Geometry check sheet. Reference: drawing and pictorial views, mm from the part's lowest x, y, z. Give positions to 0.01 mm unless a question says otherwise; leave off trailing zeros. Write each loop counter-clockwise with the first axis right and the second up, starting at its lowest first coordinate (ties: lowest second). Pieces come first, ordered by that corner, then holes. Notation, with made-up numbers: (22.25, 3) - (37.25, 3) arc R13 cw to (37.25, 17) - close; hole circle Ø5 at (23, 81.25). An arc over 180 degrees is marked (long way). Put each result on its own line as item: value.
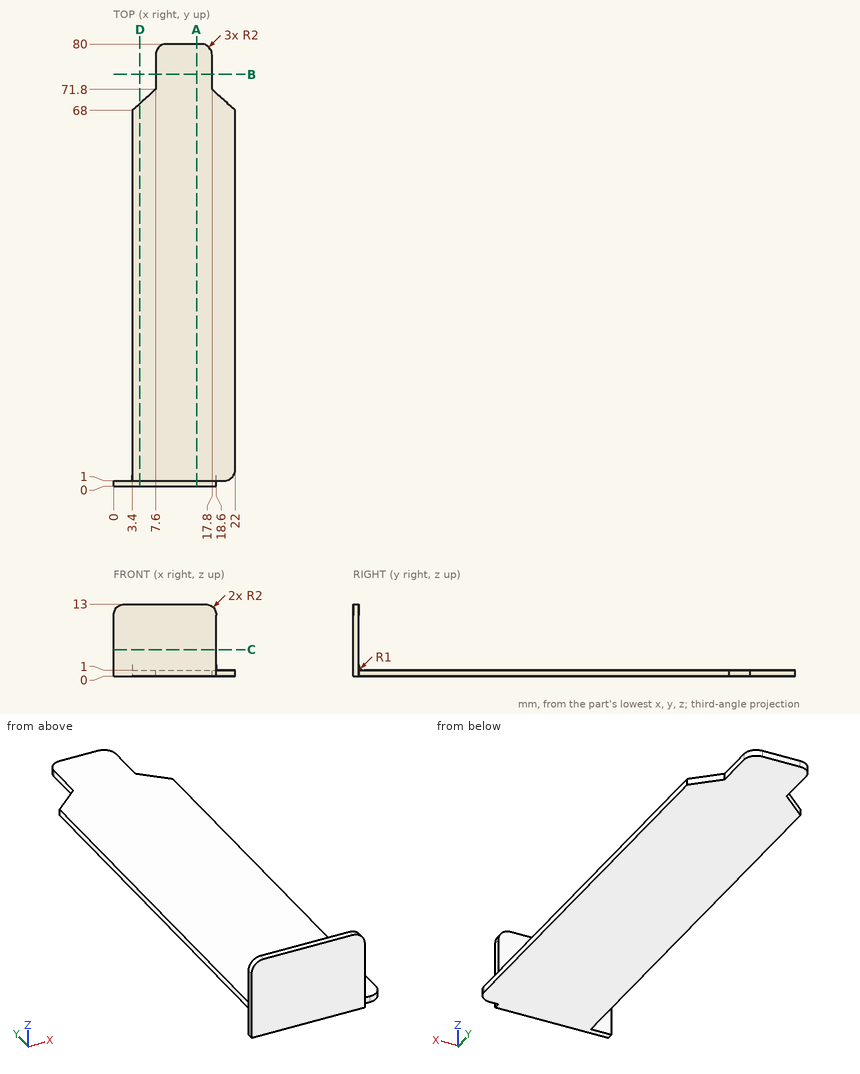
Q1. Section check D-D, the plane x = 4.75. Record the cut outline in (y, z).
Answers follow:
outline: (0, 0) - (69.22, 0) - (69.22, 1) - (2, 1) arc R1 cw to (1, 2) - (1, 13) - (0, 13) - close
Q2. Go/stop test with flat-tipped pins: pin 1 Ø1.1 at (y, z) = (75.5, 0.5) entering from -X; pin 2 Ø2 at (y, z) = (32, 1) entering from -X; pin 3 Ø5.5 at (x, y) = (13.5, 46.5) entering from +Z. Record where each tip stops, or that it passes through.
Answers follow:
pin 1: stops at x = 7.6
pin 2: stops at x = 3.4
pin 3: stops at z = 1
Q3. Section check A-A, the plane x = 15. Record the cut outline in (y, z), plus the area to 3 significant figures.
Answers follow:
outline: (0, 0) - (80, 0) - (80, 1) - (2, 1) arc R1 cw to (1, 2) - (1, 13) - (0, 13) - close
area: 92.2 mm2
Q4. Section check C-C, the plane z = 4.75. Record the cut outline in (x, y), plus the area to 3 significant figures.
Answers follow:
outline: (0, 0) - (18.6, 0) - (18.6, 1) - (0, 1) - close
area: 18.6 mm2
Q5. Section check B-B, the plane y = 74.5. Record the cut outline in (x, z).
Answers follow:
outline: (7.6, 0) - (17.8, 0) - (17.8, 1) - (7.6, 1) - close
Q6. Scan lines: line 1 along Y through (x, z) = (18.25, 2.5); line 2 along Y through (x, z) = (5.5, 1.5). Record each from-to range of solid material in increasing order.
Answers follow:
line 1: y = 0 to 1
line 2: y = 0 to 1.13
